Design review of the part built by this model. Coordinates are the model's own, in mm. Coordinates: 2 decimals unless noted, no trailing zeros. Loops run counter-clockwise (first coordinate to the right, second up) from the corner with the lowest first, then second, coordinate; pieces in that order, holes last. Notation, with made-up numbers: M -14.5,-1 L 1.5,-1 A22 cw 1.5,22 Z; hole C 39,53 d10. An arc over 180 degrees is marked long. Answer as a JSON object with one key per item and string values. Group by question number.
1. Consider section C-C (z = 0.55). State the section outline as (x, y) points, then the cut area to 3 significant figures.
2. Consider section B-B (x = 171). State the section outline as (y, z) points.
3. To check wall thickness, follow probe 1 along Y at (x, z) = (-32.5, 0.25); probe 2 along Y at (x, z) = (173.5, 1.15); probe 3 along X at (y, z) = (-437, 1.4). State the ranges of each line that lie inside material, in increasing order.
4. Consider section A-A (y = -275). State the section outline as (x, z) points, then the cut area to 3 significant figures.
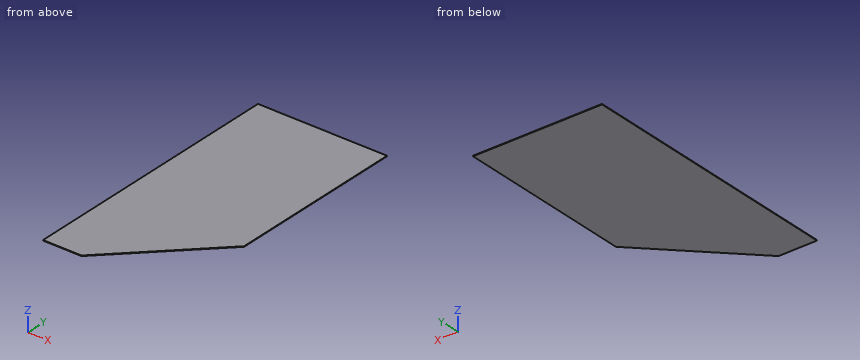
Autodesk Inventor part; units mm, degrees
ref_plane "YZ Plane" through (0, 0, 0) normal (1, 0, 0) x (0, 1, 0)
ref_plane "XZ Plane" through (0, 0, 0) normal (0, 1, 0) x (-1, 0, 0)
ref_plane "XY Plane" through (0, 0, 0) normal (0, 0, 1) x (1, 0, 0)
sketch "Sketch1" plane through (0, 0, 0) normal (0, 0, 1) x (1, 0, 0)
  line L0 (-251, -525) -> (251, -525)
  line L1 (251, -525) -> (251, 525)
  line L2 (251, 525) -> (-251, 525)
  line L3 (-251, 525) -> (-251, -525)
  line L4 (-251, -525) -> (251, 525) construction
  line L5 (251, -525) -> (-251, 525) construction
  line L6 (-101, -525) -> (251, -173)
  point P0 (0, 0)
  dimension "d0" = 502
  dimension "d1" = 1050
  dimension "d12" = 698
  dimension "d13" = 150
extrude "Plate1" add sketch "Sketch1" along normal blind 2 contours L3 L2 L1 L6 L0
sketch "Sketch2" plane through (0, 0, 0) normal (0, 0, -1) x (-1, 0, 0)
  line L0 (-231, 505) -> (-31, 505) construction
  line L1 (-31, 505) -> (-31, 485) construction
  line L2 (-31, 485) -> (-231, 485) construction
  line L3 (-231, 485) -> (-231, 505) construction
  line L4 (-251, 525) -> (251, 525)
  line L5 (-251, -173) -> (-251, 525)
  point P0 (0, 0)
  point P1 (-48, 100)
  point P2 (-251, -525)
  point P3 (-50, 98)
  dimension "d6" = 200
  dimension "d9" = 20
  dimension "d10" = 20
  dimension "d11" = 20
mark "Mark1"
equation "\"d2\" = Thickness"
equation "\"BendReliefWidth\" = Thickness"
equation "\"BendReliefDepth\" = 0.5 * Thickness"
equation "\"CornerReliefSize\" = 4 * Thickness"
equation "\"MinimumRemnant\" = 2 * Thickness"
equation "\"TransitionRadius\" = BendRadius"
equation "\"JacobiRadiusSize\" = BendRadius"
equation "\"GapSize\" = Thickness"
properties part number "TRM 016 right board main" material "AISI 304"
Findings below:
{
 "1": {"outline": "M -251,-525 L -101,-525 L 251,-173 L 251,525 L -251,525 Z", "area": "465,000 mm^2"},
 "2": {"outline": "M -253,0 L 525,0 L 525,2 L -253,2 Z"},
 "3": {"probe 1": "y = -456.5 to 525", "probe 2": "y = -250.5 to 525", "probe 3": "x = -251 to -13"},
 "4": {"outline": "M -251,0 L 149,0 L 149,2 L -251,2 Z", "area": "800 mm^2"}
}
